Source: CAD feature listing. Evaluate the final solid. Frame: model axes, mm. Face numbers are marked on the shaded views. A direction names the side the tool comes from. Coordinates: 2 decimals unless noted, no trailing zeros. Order: outer loops, then holes, each group sorted by start corner. A loop starts at its lowest first (then second) coordinate and runs counter-clockwise, first axis right, second up. Notation, with made-up numbers: (19.25, 89.5) - (78.25, 89.5) arc R33 cw to (78.25, 117.5) - close; hole circle Ø7 at (12.25, 18). An arc over 180 degrees is marked (long way). One line per question, with ' | ' between items.
from build123d import *

# Parameters (mm, degrees)
SKETCH2_R           = 2.5
BOSS_EXTRUDE1_DEPTH = 3


with BuildPart() as part:
    # Sketch2 → Boss-Extrude1 (new body)
    with BuildSketch(Plane.XY):
        with BuildLine():
            Line((34.25, 2.05625), (49.95, 2.05625))
            ThreePointArc((49.95, 2.05625), (50.126776695, 2.129473305), (50.2, 2.30625))
            Line((50.2, 2.30625), (50.2, 5.05625))
            Line((50.2, 5.05625), (53.85, 5.05625))
            ThreePointArc((53.85, 5.05625), (54.026776695, 5.129473305), (54.1, 5.30625))
            Line((54.1, 5.30625), (54.1, 8.025))
            Line((54.1, 8.025), (56.85, 8.025))
            ThreePointArc((56.85, 8.025), (57.026776695, 8.098223305), (57.1, 8.275))
            Line((57.1, 8.275), (57.1, 12.975))
            ThreePointArc((57.1, 12.975), (57.026776695, 13.151776695), (56.85, 13.225))
            Line((56.85, 13.225), (54.1, 13.225))
            Line((54.1, 13.225), (54.1, 15.94375))
            ThreePointArc((54.1, 15.94375), (54.026776695, 16.120526695), (53.85, 16.19375))
            Line((53.85, 16.19375), (50.2, 16.19375))
            Line((50.2, 16.19375), (50.2, 18.94375))
            ThreePointArc((50.2, 18.94375), (50.126776695, 19.120526695), (49.95, 19.19375))
            Line((49.95, 19.19375), (34.25, 19.19375))
            ThreePointArc((34.25, 19.19375), (34.073223305, 19.120526695), (34, 18.94375))
            Line((34, 18.94375), (34, 16.19375))
            Line((34, 16.19375), (22.7, 16.19375))
            Line((22.7, 16.19375), (22.7, 18.94375))
            ThreePointArc((22.7, 18.94375), (22.626776695, 19.120526695), (22.45, 19.19375))
            Line((22.45, 19.19375), (6.75, 19.19375))
            ThreePointArc((6.75, 19.19375), (6.573223305, 19.120526695), (6.5, 18.94375))
            Line((6.5, 18.94375), (6.5, 16.19375))
            Line((6.5, 16.19375), (2.85, 16.19375))
            ThreePointArc((2.85, 16.19375), (2.673223305, 16.120526695), (2.6, 15.94375))
            Line((2.6, 15.94375), (2.6, 13.225))
            Line((2.6, 13.225), (-0.15, 13.225))
            ThreePointArc((-0.15, 13.225), (-0.326776695, 13.151776695), (-0.4, 12.975))
            Line((-0.4, 12.975), (-0.4, 8.275))
            ThreePointArc((-0.4, 8.275), (-0.326776695, 8.098223305), (-0.15, 8.025))
            Line((-0.15, 8.025), (2.6, 8.025))
            Line((2.6, 8.025), (2.6, 5.30625))
            ThreePointArc((2.6, 5.30625), (2.673223305, 5.129473305), (2.85, 5.05625))
            Line((2.85, 5.05625), (6.5, 5.05625))
            Line((6.5, 5.05625), (6.5, 2.30625))
            ThreePointArc((6.5, 2.30625), (6.573223305, 2.129473305), (6.75, 2.05625))
            Line((6.75, 2.05625), (22.45, 2.05625))
            ThreePointArc((22.45, 2.05625), (22.626776695, 2.129473305), (22.7, 2.30625))
            Line((22.7, 2.30625), (22.7, 5.05625))
            Line((22.7, 5.05625), (34, 5.05625))
            Line((34, 5.05625), (34, 2.30625))
            ThreePointArc((34, 2.30625), (34.073223305, 2.129473305), (34.25, 2.05625))
        make_face()
        with Locations((17.1, 9.15625)):
            Circle(SKETCH2_R, mode=Mode.SUBTRACT)
        with Locations((41.1, 9.15625)):
            Circle(SKETCH2_R, mode=Mode.SUBTRACT)
    extrude(amount=BOSS_EXTRUDE1_DEPTH)


solid = part.part
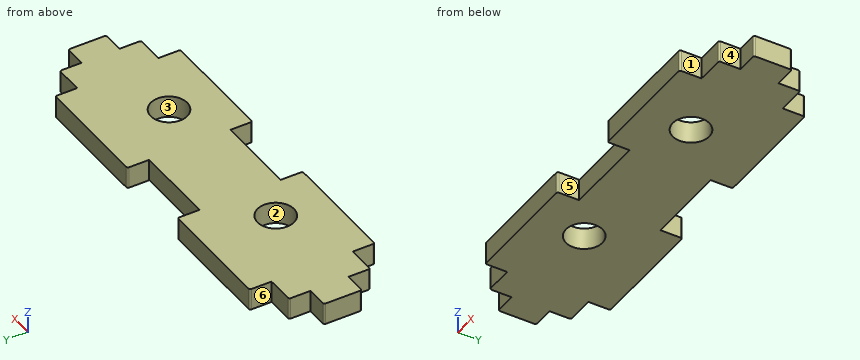
(1) Cut plane C-C (z = 2.1). State how many separate pieces and enclosed holes the cut face has, and give its area (3 significant figures).
Taken from the geometry:
separate pieces: 1 | enclosed holes: 2 | area: 760 mm²
(2) Pin query (flat end, axial travel): P1, Ø0.8, axis at x = 56, z = 1, coming from the +Y side (3 decimals); P2, Ø1, axis at x = 30, z = 2, coming from the +Y side; P3, Ø4, axis at x = 17.1, y = 9.16, coming from the -Z side; P4, Ø0.8, axis at y = 4, z = 1, coming from the +X side. Return the tip coordinate at first contact, or that it passes through.
Taken from the geometry:
P1: stops at y = 13.225 | P2: stops at y = 16.19 | P3: passes through | P4: stops at x = 50.2
(3) Cut plane B-B (y = 17). Return the cut outline in (x, z), and give its area (3 significant figures).
Taken from the geometry:
outline: (6.5, 0) - (22.7, 0) - (22.7, 3) - (6.5, 3) - close; (34, 0) - (50.2, 0) - (50.2, 3) - (34, 3) - close | area: 97.2 mm²
(4) Cut plane A-A (x = 17.1). Return the cut outline in (y, z), and give its area (3 significant figures).
Taken from the geometry:
outline: (2.06, 0) - (6.66, 0) - (6.66, 3) - (2.06, 3) - close; (11.66, 0) - (19.19, 0) - (19.19, 3) - (11.66, 3) - close | area: 36.4 mm²
(5) Material intervals for L1, parallel to Y at x = 41.1, z = 2.3; L2, parallel to X at y = 7, z = 2.7; L3, parallel to X at y = 3.5, z = 2.9, sorted ascending. Write a range as from..to.
Taken from the geometry:
L1: y = 2.06..6.66, 11.66..19.19 | L2: x = 2.6..15.83, 18.37..39.83, 42.37..54.1 | L3: x = 6.5..22.7, 34..50.2
(6) Pull-direction query (Y, two-part tool) for the marked faces 1, 2 and 3; classes: pulls with the +Y half, pulls with the -Y half, needs draft (parallel to the pull), parting line crosses it, or undercut.
Taken from the geometry:
face 1: needs draft | face 2: undercut | face 3: undercut
(7) Set-up query: the marked faces 4, 5 and 6. Return all of +Z, -Z, +X, -X, +Y, -Y with unobstructed straight access to the full face (end or side cutting, diameter ignored); none if empty.
Taken from the geometry:
face 4: +Z, -Z, +X, -Y | face 5: +Z, -Z, -Y | face 6: +Z, -Z, -X, +Y
